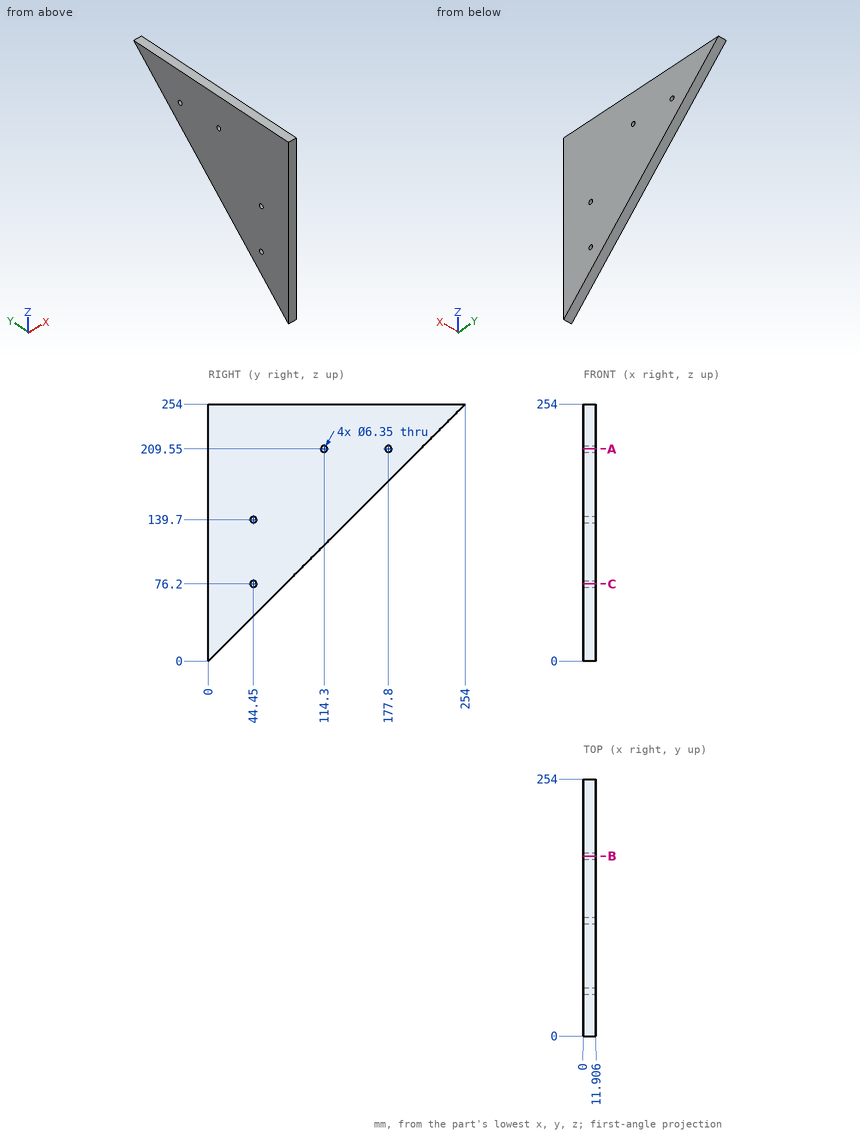
Here's the drawing with two shaded views (mm, measured from the low corner). I have some questions. Give positions to 0.01 mm unless a question says otherwise; leave off trailing zeros. Write each loop counter-clockwise with the first axis right and the second up, starting at its lowest first coordinate (ties: lowest second). Pieces come first, ordered by that corner, then holes. Notation, with made-up numbers: (28.5, 67.25) - (86.5, 67.25) arc R28 ccw to (86.5, 105.25) - close; hole circle Ø4 at (37.5, 1). An arc over 180 degrees is marked (long way). One line per item, written item: value. Start each with the question number.
Item 1: Imagine slicing it at C-C, the plane z = 76.2. List the corners of the cut face in (x, y) for me (1 decimal).
Item 2: Imagine slicing it at B-B, the plane y = 177.8. List the corners of the cut face in (x, z) for me (1 decimal).
Item 3: Please list where these lines run through material, in increasing order: line 1 (Y direction, x = 5.75, z = 139.7) (1 decimal); line 2 (Z direction, x = 5, y = 228.5); line 3 (Y direction, x = 8.5, z = 224). Write a range as from..to.
Item 4: Imagine slicing it at A-A, the plane z = 209.55. Give the number of separate pieces and of enclosed holes in the cut face, and give its area (3 significant figures).
Item 5: I'm going to push flat-ended pins straight in: pin 1 (3 mm diameter, centred on x = 6, y = 207, fed in from -Z); pin 2 (6 mm diameter, centred on x = 5, z = 60, fed in from +Y). Where does each tip first touch, or does it pass through?
Geometry says:
1. outline: (0, 0) - (11.9, 0) - (11.9, 41.3) - (0, 41.3) - close; (0, 47.6) - (11.9, 47.6) - (11.9, 76.2) - (0, 76.2) - close
2. outline: (0, 177.8) - (11.9, 177.8) - (11.9, 206.4) - (0, 206.4) - close; (0, 212.7) - (11.9, 212.7) - (11.9, 254) - (0, 254) - close
3. line 1: 0..41.3, 47.6..139.7
3. line 2: 228.5..254
3. line 3: 0..224
4. separate pieces: 3
4. enclosed holes: 0
4. area: 2,340 mm^2
5. pin 1: z = 205.5
5. pin 2: y = 63
